Verification items for the finished model (mm, model axes). A direction names the side the tool comes from. Give positions to 0.01 mm unless a question says otherwise; leave off trailing zeros. Order: outer loops, then holes, each group sorted by start corner. A loop starts at its lowest first (then second) coordinate and runs counter-clockwise, first axis right, second up.
Autodesk Inventor part; units mm, degrees
ref_plane "YZ Plane" through (0, 0, 0) normal (1, 0, 0) x (0, 1, 0)
ref_plane "XZ Plane" through (0, 0, 0) normal (0, 1, 0) x (-1, 0, 0)
ref_plane "XY Plane" through (0, 0, 0) normal (0, 0, 1) x (1, 0, 0)
sketch "スケッチ1" plane through (0, 0, 0) normal (0, 0, 1) x (1, 0, 0)
  line L0 (0, 0) -> (50, 0)
  line L1 (50, 0) -> (50, 50)
  line L2 (50, 50) -> (0, 50)
  line L3 (0, 50) -> (0, 0)
  line L4 (2, 48) -> (48, 48)
  line L5 (48, 48) -> (48, 2)
  line L6 (48, 2) -> (2, 2)
  line L7 (2, 2) -> (2, 48)
  dimension "d0" = 50
  dimension "d1" = 2
extrude "押し出し1" add sketch "スケッチ1" along normal blind 50
sketch "スケッチ2" plane through (0, 50, 0) normal (0, 1, 0) x (1, 0, 0)
  point P0 (0, 0)
sketch "スケッチ3" plane through (50, 0, 0) normal (1, 0, 0) x (0, 0, -1)
  line L0 (0, 0) -> (0, 50)
  line L1 (0, 50) -> (-50, 50)
  line L2 (-50, 0) -> (-50, 50)
  line L3 (0, 0) -> (-50, 0)
  line L4 (-50, 10) -> (0, 10) construction
  line L5 (-25, 50) -> (-25, 0) construction
  point P0 (-44, 10)
  point P1 (-6, 10)
  dimension "d5" = 6
  dimension "d21" = 10
hole "穴1" at (50, 10, 44) at (50, 10, 6) direction (-1, 0, 0) diameter 4.5 end through all
sketch "スケッチ4" plane through (0, 0, 0) normal (0, -1, 0) x (1, 0, 0)
  line L0 (0, 0) -> (50, 0)
  line L1 (50, 0) -> (50, 50)
  line L2 (0, 50) -> (50, 50)
  line L3 (0, 0) -> (0, 50)
  line L4 (25, 50) -> (25, 0) construction
  point P0 (25, 32)
  dimension "d20" = 18
hole "穴2" at (25, 0, 32) direction (0, 1, 0) diameter 22 depth 2
properties part number "ankle" material "アルミニウム 6061"
(1) Section check B-B, the plane x = 25. Enter the section's corners in (y, z).
Solved:
outline: (0, 0) - (2, 0) - (2, 21) - (0, 21) - close; (0, 43) - (2, 43) - (2, 50) - (0, 50) - close; (48, 0) - (50, 0) - (50, 50) - (48, 50) - close
(2) Go/stop test with a flat-tipped pin: pin 1 (17.5 mm diameter, centred on x = 25, z = 32, fed in from -Y). Record where the tip stops, or that it passes through.
Solved:
pin 1: stops at y = 48
(3) Set-up check for faces 1 (the cylindrical face through (34.759, 1.014, 26.924)), 2 (the flat face through (48, 25, 25)), 3 (the flat face through (23, 1, 50)): record each of +Z, -Z, +X, -X, +Y, -Y from which the full face is reachable in a straight line by a thin tool's end or side.
Solved:
face 1: -Y
face 2: +Z, -Z
face 3: +Z, +X, -X, +Y, -Y
(4) Section check A-A, the plane y = 37. Enter the section's corners in (x, z).
Solved:
outline: (0, 0) - (2, 0) - (2, 50) - (0, 50) - close; (48, 0) - (50, 0) - (50, 50) - (48, 50) - close
(5) Scan lines: line 1 (Z direction, x = 48.5, y = 10); line 2 (X direction, y = 20.5, z = 43.5). Record each from-to range of solid material in increasing order.
Solved:
line 1: z = 0 to 3.75, 8.25 to 41.75, 46.25 to 50
line 2: x = 0 to 2, 48 to 50
(6) Release check for a two-part mould opening along X. For faces 4 (the flat face through (25, 2, 19)), 5 (the cylindrical face through (48.986, 8.103, 4.79)), 6 (the flat face through (0, 25, 25)) record: pulls with the +X half, pulls with the -X half, needs draft (parallel to the pull), parting line crosses it, or undercut.
Solved:
face 4: undercut
face 5: needs draft
face 6: pulls with the -X half
(7) Section check C-C, the plane z = 6. Enter the section's corners in (x, y), then the cut area to 3 significant figures.
Solved:
outline: (0, 0) - (50, 0) - (50, 7.75) - (48, 7.75) - (48, 2) - (2, 2) - (2, 7.75) - (0, 7.75) - close; (0, 12.25) - (2, 12.25) - (2, 48) - (48, 48) - (48, 12.25) - (50, 12.25) - (50, 50) - (0, 50) - close
area: 366 mm2
